Autodesk Fusion 360 part; units mm, degrees
sketch "Sketch1" plane through (0, 0, 0) normal (0, 0, 1) x (1, 0, 0)
  line L0 (-25, 0) -> (-15, 0)
  line L1 (-15, 0) -> (-15, 5)
  line L2 (-15, 5) -> (-10, 5)
  line L3 (-10, 5) -> (-10, 10)
  line L4 (-10, 10) -> (-5, 10)
  line L5 (-5, 10) -> (-5, 15)
  line L6 (-5, 15) -> (-1.7883, 15)
  line L7 (-1.7883, 15) -> (0, 15)
  line L8 (0, 15) -> (0, 55)
  line L9 (0, 55) -> (-5, 55)
  line L10 (-5, 55) -> (-5, 60)
  line L11 (-5, 60) -> (-10, 60)
  line L12 (-10, 60) -> (-10, 65)
  line L13 (-10, 65) -> (-15, 65)
  line L14 (-15, 65) -> (-15, 70)
  line L15 (-15, 70) -> (-80, 70)
  line L16 (-80, 70) -> (-80, 65)
  line L17 (-80, 65) -> (-85, 65)
  line L18 (-85, 65) -> (-85, 60)
  line L19 (-85, 60) -> (-90, 60)
  line L20 (-90, 60) -> (-90, 55)
  line L21 (-90, 55) -> (-95, 55)
  line L22 (-95, 55) -> (-95, 15)
  line L23 (-95, 15) -> (-90, 15)
  line L24 (-90, 15) -> (-90, 10)
  line L25 (-90, 10) -> (-85, 10)
  line L26 (-85, 10) -> (-85, 5)
  line L27 (-85, 5) -> (-80, 5)
  line L28 (-80, 5) -> (-80, 0)
  line L29 (-80, 0) -> (-25, 0)
extrude "Extrude1" add sketch "Sketch1" along normal blind 5
hole "Hole1" at (-75.2055, 57.6429, 5) direction (0, 0, -1) diameter 10 depth 30 tip angle 118
sketch "Sketch2" plane through (0, 0, 5) normal (0, 0, 1) x (-1, 0, 0)
  circle A0 centre (75.2055, -57.6429) radius 5
  line L0 (80, 0) -> (15, 0)
  line L1 (15, 0) -> (15, -5)
  line L2 (15, -5) -> (10, -5)
  line L3 (10, -5) -> (10, -10)
  line L4 (10, -10) -> (5, -10)
  line L5 (5, -10) -> (5, -15)
  line L6 (5, -15) -> (0, -15)
  line L7 (0, -15) -> (0, -55)
  line L8 (0, -55) -> (5, -55)
  line L9 (5, -55) -> (5, -60)
  line L10 (5, -60) -> (10, -60)
  line L11 (10, -60) -> (10, -65)
  line L12 (10, -65) -> (15, -65)
  line L13 (15, -65) -> (15, -70)
  line L14 (15, -70) -> (80, -70)
  line L15 (80, -70) -> (80, -65)
  line L16 (80, -65) -> (85, -65)
  line L17 (85, -65) -> (85, -60)
  line L18 (85, -60) -> (90, -60)
  line L19 (90, -60) -> (90, -55)
  line L20 (90, -55) -> (95, -55)
  line L21 (95, -55) -> (95, -15)
  line L22 (95, -15) -> (90, -15)
  line L23 (90, -15) -> (90, -10)
  line L24 (90, -10) -> (85, -10)
  line L25 (85, -10) -> (85, -5)
  line L26 (85, -5) -> (80, -5)
  line L27 (80, -5) -> (80, 0)
  line L28 (80, -45) -> (80, -21.0556)
  line L29 (80, -21.0556) -> (65, -21.0556)
  line L30 (65, -21.0556) -> (65, -43.5828)
  line L31 (65, -43.5828) -> (65, -45)
  line L32 (65, -45) -> (70, -45)
  line L33 (70, -45) -> (70, -30)
  line L34 (70, -30) -> (75, -30)
  line L35 (75, -30) -> (75, -45)
  line L36 (75, -45) -> (80, -45)
  line L37 (60, -45) -> (45, -45)
  line L38 (45, -45) -> (45, -40)
  line L39 (45, -40) -> (55, -40)
  line L40 (55, -40) -> (55, -35)
  line L41 (55, -35) -> (45, -35)
  line L42 (45, -35) -> (45, -25)
  line L43 (45, -25) -> (45, -20)
  line L44 (45, -20) -> (60, -20)
  line L45 (60, -20) -> (60, -25)
  line L46 (60, -25) -> (50, -25)
  line L47 (50, -25) -> (50, -30)
  line L48 (50, -30) -> (60, -30)
  line L49 (60, -30) -> (60, -45)
  line L50 (40, -45) -> (40, -20)
  line L51 (40, -20) -> (25, -20)
  line L52 (25, -20) -> (25, -45)
  line L53 (25, -45) -> (30, -45)
  line L54 (30, -45) -> (30, -30)
  line L55 (30, -30) -> (35, -30)
  line L56 (35, -30) -> (35, -45)
  line L57 (35, -45) -> (40, -45)
  line L58 (20, -45) -> (5, -45)
  line L59 (5, -45) -> (12.5, -25.2503)
  line L60 (12.5, -25.2503) -> (20, -45)
  circle A1 centre (12.4062, -18.7252) radius 4.684
  line L61 (53.32, -17.4727) -> (55, -15)
  line L62 (55, -15) -> (51.9633, -15)
  line L63 (51.9633, -15) -> (55, -10.5305)
  line L64 (55, -10.5305) -> (50, -15)
  line L65 (50, -15) -> (51.9633, -16.3339)
  line L66 (51.9633, -16.3339) -> (51.9633, -18.151)
  line L67 (51.9633, -18.151) -> (53.32, -17.4727)
extrude "Extrude2" add sketch "Sketch2" along normal blind 5 contours L28 L29 L30 L31 L32 L33 L34 L35 L36 | L37 L38 L39 L40 L41 L42 L43 L44 L45 L46 L47 L48 L49 | L50 L51 L52 L53 L54 L55 L56 L57 | L58 L59 L60 | A1 | L61 L62 L63 L64 L65 L66 L67
Work out the finished part from the listing and answer in its coordinate system (mm). A direction names the side the tool comes from. Give positions to 0.01 mm unless a question says otherwise; leave off trailing zeros. Loops run counter-clockwise (first coordinate to the right, second up) from the corner with the lowest first, then second, coordinate; pieces in that order, holes last. Notation, with made-up numbers: (4.25, -16.5) -> (53.25, -16.5) arc R28 ccw to (53.25, 21.5) -> close; hole circle Ø11 at (54, -25). An arc over 180 degrees is marked (long way). Use a Markdown table: item, result. Add a question column.
1. Section D-D on y = 41 is taken. Determine the outline of the cut face in (x, z), and give its area (3 significant figures).
2. Section A-A on x = -38 is taken. Determine the outline of the cut face in (y, z).
3. For faces 4 (the flat face through (-10, 62, 2)), 5 (the flat face through (-80, 68, 2)), 6 (the flat face through (-15, 2, 2)), 7 (the flat face through (-40, 33, 7)), determine the directions among +Z, -Z, +X, -X, +Y, -Y from which every point of the face is accessible in a straight line to the end or side of a thin tool.
4. Section B-B on y = 58 is taken. Determine the outline of the cut face in (x, z), and give its area (3 significant figures).
5. Find the intervals of material crossed by probe 1 along X at (y, z) = (29, 5.25); probe 2 along Y at (x, z) = (-4, 1); probe 3 along Y at (x, z) = (-8.5, 4.25), in increasing order.
6. Flat-ended cylindrical pins translate along their axes: pin 1 Ø5.5 at (y, z) = (41, 7) entering from -X; pin 2 Ø2 at (x, z) = (-12.5, 2.5) entering from -Y; pin 3 Ø0.9 at (y, z) = (17, 7) entering from +X; pin 4 Ø4 at (y, z) = (61.5, 3.5) entering from -X. Find the tip coordinate at first contact, or state that the pin passes through.
7. Determine the mould class of faces 1 (the flat face through (-80, 3, 2)), 2 (the flat face through (-15, 67, 2)), 3 (the flat face through (-32, 30, 7)) for opening direction X: released by +X, released by -X, zero draft, split by the parting line, or undercut.
Results below:
| question | item | result |
|---|---|---|
| 1 | outline | (-95, 0) -> (0, 0) -> (0, 5) -> (-6.52, 5) -> (-6.52, 10) -> (-18.48, 10) -> (-18.48, 5) -> (-25, 5) -> (-25, 10) -> (-30, 10) -> (-30, 5) -> (-35, 5) -> (-35, 10) -> (-40, 10) -> (-40, 5) -> (-45, 5) -> (-45, 10) -> (-60, 10) -> (-60, 5) -> (-65, 5) -> (-65, 10) -> (-70, 10) -> (-70, 5) -> (-75, 5) -> (-75, 10) -> (-80, 10) -> (-80, 5) -> (-95, 5) -> close |
| 1 | area | 710 mm^2 |
| 2 | outline | (0, 0) -> (70, 0) -> (70, 5) -> (45, 5) -> (45, 10) -> (20, 10) -> (20, 5) -> (0, 5) -> close |
| 3 | face 4 | +Z, -Z, +X, +Y |
| 3 | face 5 | +Z, -Z, -X, +Y |
| 3 | face 6 | +Z, -Z, +X, -Y |
| 3 | face 7 | +Z, +Y, -Y |
| 4 | outline | (-90, 0) -> (-80.19, 0) -> (-80.19, 5) -> (-90, 5) -> close; (-70.22, 0) -> (-5, 0) -> (-5, 5) -> (-70.22, 5) -> close |
| 4 | area | 375 mm^2 |
| 5 | probe 1 | x = -80 to -65, -50 to -45, -40 to -25, -13.92 to -11.08 |
| 5 | probe 2 | y = 15 to 55 |
| 5 | probe 3 | y = 10 to 60 |
| 6 | pin 1 | stops at x = -95 |
| 6 | pin 2 | stops at y = 5 |
| 6 | pin 3 | stops at x = -7.9 |
| 6 | pin 4 | stops at x = -90 |
| 7 | face 1 | released by -X |
| 7 | face 2 | released by +X |
| 7 | face 3 | undercut |
